For this review, take the finished solid that the model builds, in its own axes (mm). A direction names the side the tool comes from. Give positions to 0.01 mm unless a question says otherwise; leave off trailing zeros. Loops run counter-clockwise (first coordinate to the right, second up) from the corner with the lowest first, then second, coordinate; pieces in that order, holes last.
```python
from build123d import *

# Parameters (mm, degrees)
SKETCH1_W           = 140
SKETCH1_H           = 140
BOSS_EXTRUDE1_DEPTH = 5
CUT_EXTRUDE2_DEPTH  = 5
SKETCH3_W           = 26
SKETCH3_H           = 26
CUT_EXTRUDE3_DEPTH  = 5
SKETCH5_R           = 1.525
CUT_EXTRUDE5_DEPTH  = 5
SKETCH7_W           = 0.499998827
SKETCH7_H           = 0.5
SKETCH7_W_2         = 0.5
CUT_EXTRUDE6_DEPTH  = 5


with BuildPart() as part:
    # Sketch1 → Boss-Extrude1 (new body)
    with BuildSketch(Plane(origin=(0, 0, 0), x_dir=(1, 0, 0), z_dir=(0, 1, 0))):
        Rectangle(SKETCH1_W, SKETCH1_H)
    extrude(amount=BOSS_EXTRUDE1_DEPTH)

    # Sketch2 → Cut-Extrude2 (cut)
    with BuildSketch(Plane(origin=(0, 5, 0), x_dir=(1, 0, 0), z_dir=(0, 1, 0))):
        Polygon((-13, 13), (13, 13), (13, 13.5), (13.5, 13.5), (13.5, 42.495538118), (-13.499998827, 42.495538118), (-13.499998827, 13.5), (-13, 13.5), align=None)
        Polygon((-13.499998827, -13), (-13, -13), (-13, 13), (-13.499998827, 13), (-13.499998827, 13.5), (-42, 13.5), (-42, -13.5), (-13.499998827, -13.5), align=None)
        Polygon((13, 13), (13, -13), (13.5, -13), (13.5, -13.5), (42, -13.5), (42, 13.5), (13.5, 13.5), (13.5, 13), align=None)
        Polygon((13.5, -13.5), (13, -13.5), (13, -13), (-13, -13), (-13, -13.5), (-13.499998827, -13.5), (-13.499998827, -42.495538118), (13.5, -42.495538118), align=None)
    extrude(amount=-CUT_EXTRUDE2_DEPTH, mode=Mode.SUBTRACT)

    # Sketch3 → Cut-Extrude3 (cut)
    with BuildSketch(Plane(origin=(0, 5, 0), x_dir=(1, 0, 0), z_dir=(0, 1, 0))):
        Rectangle(SKETCH3_W, SKETCH3_H)
    extrude(amount=-CUT_EXTRUDE3_DEPTH, mode=Mode.SUBTRACT)

    # Sketch5 → Cut-Extrude5 (cut)
    with BuildSketch(Plane(origin=(0, 5, 0), x_dir=(1, 0, 0), z_dir=(0, 1, 0))):
        with Locations(Location((-56.8, -19.996300578, 0), (0, 0, 270))):
            Circle(SKETCH5_R)
        with Locations(Location((-19.95, -56.803699422, 0), (0, 0, 270))):
            Circle(SKETCH5_R)
        with Locations(Location((19.95, 56.803699422, 0), (0, 0, 270))):
            Circle(SKETCH5_R)
        with Locations(Location((56.8, 19.996300578, 0), (0, 0, 270))):
            Circle(SKETCH5_R)
    extrude(amount=-CUT_EXTRUDE5_DEPTH, mode=Mode.SUBTRACT)

    # Sketch7 → Cut-Extrude6 (cut)
    with BuildSketch(Plane(origin=(0, 5, 0), x_dir=(1, 0, 0), z_dir=(0, 1, 0))):
        with Locations((-13.249999413, -13.25)):
            Rectangle(SKETCH7_W, SKETCH7_H)
        with Locations((-13.249999413, 13.25)):
            Rectangle(SKETCH7_W, SKETCH7_H)
        with Locations((13.25, 13.25)):
            Rectangle(SKETCH7_W_2, SKETCH7_H)
        with Locations((13.25, -13.25)):
            Rectangle(SKETCH7_W_2, SKETCH7_H)
    extrude(amount=-CUT_EXTRUDE6_DEPTH, mode=Mode.SUBTRACT)


solid = part.part
```
Item 1: Tool access review of faces 5 (the flat face through (28, 3, 13.5)), 6 (the flat face through (15, 0, -17)): name each direction out of +Z, -Z, +X, -X, +Y, -Y from which nothing blocks a thin tool from reaching the whole face with its end or side.
Answer:
face 5: +Y, -Y
face 6: +Z, -Z, +X, -X, -Y
Item 2: Take a section at A-A on x = -3. Give the boundary of the cut face in (y, z).
Answer:
outline: (0, -70) - (5, -70) - (5, -42.5) - (0, -42.5) - close; (0, 42.5) - (5, 42.5) - (5, 70) - (0, 70) - close
Item 3: For L1, parallel to X at y = 4.6, z = 16; L2, parallel to X at y = 1.5, z = 57; L3, parallel to Z at x = -4, y = 0.9, list the stretches that pass through material, from the lowest coordinate up.
Answer:
L1: x = -70 to -13.5, 13.5 to 70
L2: x = -70 to -21.46, -18.44 to 70
L3: z = -70 to -42.5, 42.5 to 70
Item 4: The part is to be moulded in two halves that separate along X. For faces 1 (the flat face through (-13.5, 3, -28)), 2 (the flat face through (-1, 2, 70)), 3 (the flat face through (70, 2, 1)), 4 (the cylindrical face through (57.83, 2.54, -21.12)), say which applies: released by +X, released by -X, zero draft, split by the parting line, or undercut.
Answer:
face 1: undercut
face 2: zero draft
face 3: released by +X
face 4: undercut
Item 5: Take a section at B-B on z = 33.5. Give the boundary of the cut face in (x, y), and give its area (3 significant figures).
Answer:
outline: (-70, 0) - (-13.5, 0) - (-13.5, 5) - (-70, 5) - close; (13.5, 0) - (70, 0) - (70, 5) - (13.5, 5) - close
area: 565 mm2
Item 6: Take a section at C-C on y = 3.9. Give the boundary of the cut face in (x, z) (3 decimals).
Answer:
outline: (-70, -70) - (70, -70) - (70, 70) - (-70, 70) - close; hole circle Ø3.05 at (-56.8, 19.996); hole (-42, -13.5) - (-13.5, -13.5) - (-13.5, -42.496) - (13.5, -42.496) - (13.5, -13.5) - (42, -13.5) - (42, 13.5) - (13.5, 13.5) - (13.5, 42.496) - (-13.5, 42.496) - (-13.5, 13.5) - (-42, 13.5) - close; hole circle Ø3.05 at (-19.95, 56.804); hole circle Ø3.05 at (19.95, -56.804); hole circle Ø3.05 at (56.8, -19.996)
Item 7: Clearance check with flat-ended pins moving along their axes: pin 1 Ø5 at (x, z) = (19.95, -56.8) entering from -Y; pin 2 Ø1.8 at (x, z) = (-56.8, 20) entering from +Y. State where each tip first meets the part, or that it passes through.
Answer:
pin 1: stops at y = 0
pin 2: passes through
